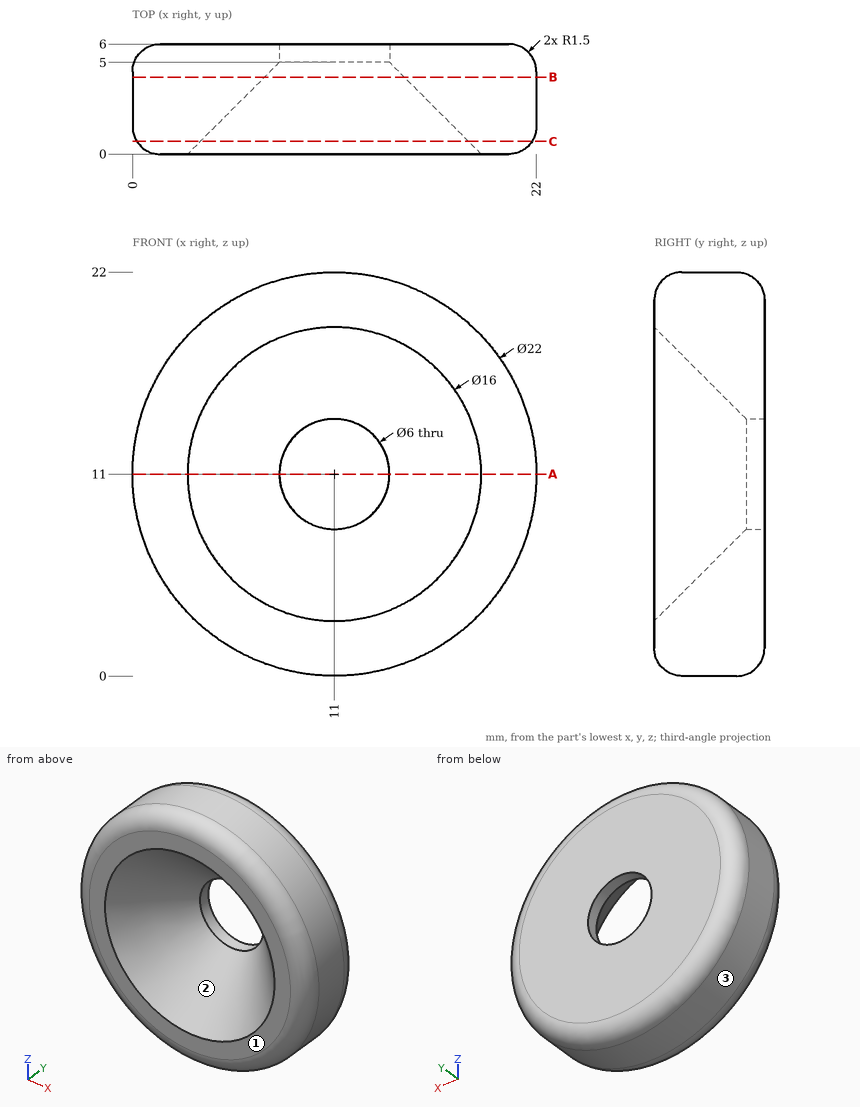
Part print with two shaded views. Sizes in mm from the minimum x, y, z corner. Coordinates: 2 decimals unless noted, no trailing zeros. Write each loop counter-clockwise with the first axis right and the second up, starting at its lowest first coordinate (ties: lowest second). Pieces come first, ordered by that corner, then holes. Notation, with made-up numbers: (72, 1) -> (86, 1) arc R23 cw to (86, 17) -> close; hole circle Ø2 at (65.5, 72). An arc over 180 degrees is marked (long way). Return JSON: item names as keys, results as strings. Group by question number.
Q1. Cut at C-C, the plane y = 0.7. Give the cut face in (x, z), then the cut area to 3 significant figures.
Q2. Cut at A-A, the plane z = 11. Give the cut face in (x, y), then the cut area to 3 significant figures.
Q3. Cut at B-B, the plane y = 4.2. Give the cut face in (x, z).
Q4. Flat gauge pins, fed straight in: pin 1 (8 mm diameter, centred on x = 11, z = 11, fed in from +Y); pin 2 (3 mm diameter, centred on x = 16.5, y = 0.5, fed in from +Z); pin 3 (3 mm diameter, centred on x = 14, y = 3, fed in from -Z). Where does each tip first touch, or does it go through?
Q5. Drill centre lines: line 1 (Z direction, x = 11.75, y = 4.8); line 2 (X direction, y = 5.25, z = 11); line 3 (X direction, y = 5.55, z = 11). Where is each one in solid material? Low to high.
Q6. Pull direction X, two halves, no side cores. Call the marked faces 1, 2 and 3: released by +X, released by -X, zero draft, split by the parting line, or undercut.
Returned:
{
 "1": {"outline": "circle Ø21.54 at (11, 11); hole circle Ø14.6 at (11, 11)", "area": "197 mm2"},
 "2": {"outline": "(0, 1.5) arc R1.5 ccw to (1.5, 0) -> (3, 0) -> (8, 5) -> (8, 6) -> (1.5, 6) arc R1.5 ccw to (0, 4.5) -> close; (14, 5) -> (19, 0) -> (20.5, 0) arc R1.5 ccw to (22, 1.5) -> (22, 4.5) arc R1.5 ccw to (20.5, 6) -> (14, 6) -> close", "area": "69.1 mm2"},
 "3": {"outline": "circle Ø22 at (11, 11); hole circle Ø7.6 at (11, 11)"},
 "4": {"pin 1": "stops at y = 6", "pin 2": "stops at z = 21.14", "pin 3": "stops at z = 0.1"},
 "5": {"line 1": "z = 0.06 to 7.89, 14.11 to 21.94", "line 2": "x = 0.2 to 8, 14 to 21.8", "line 3": "x = 0.43 to 8, 14 to 21.57"},
 "6": {"face 1": "zero draft", "face 2": "undercut", "face 3": "split by the parting line"}
}
